Geometry: final body of the model. Coordinates: model frame, mm. A direction names the side the tool comes from. Coordinates: 2 decimals unless noted, no trailing zeros. Write each loop counter-clockwise with the first axis right and the second up, starting at its lowest first coordinate (ties: lowest second). Pieces come first, ordered by that corner, then holes.
from build123d import *

# Parameters (mm, degrees)
BOSS_EXTRUDE1_DEPTH = 2
FILLET1_R           = 0.5
SKETCH2_R           = 9
BOSS_EXTRUDE2_DEPTH = 1
SKETCH3_R           = 8.5
BOSS_EXTRUDE3_DEPTH = 4
CUT_EXTRUDE1_DEPTH  = 16.375249198


with BuildPart() as part:
    # Sketch1 → Boss-Extrude1 (new body)
    with BuildSketch(Plane(origin=(0, 31, 0), x_dir=(1, 0, 0), z_dir=(0, 1, 0))):
        Polygon((0, 10.392304845), (-9, 5.196152423), (-9, -5.196152423), (0, -10.392304845), (9, -5.196152423), (9, 5.196152423), align=None)
    extrude(amount=BOSS_EXTRUDE1_DEPTH)

    # Fillet1
    fillet1_edges = [part.edges().sort_by_distance(p)[0] for p in [
        (9, 32, -5.196152423),
        (9, 32, 5.196152423),
        (0, 32, 10.392304845),
        (-9, 32, 5.196152423),
        (-9, 32, -5.196152423),
        (0, 32, -10.392304845),
    ]]
    fillet(fillet1_edges, radius=FILLET1_R)

    # Sketch2 → Boss-Extrude2 (add)
    with BuildSketch(Plane(origin=(0, 33, 0), x_dir=(1, 0, 0), z_dir=(0, 1, 0))):
        with Locations(Location((0, 0, 0), (0, 0, 60))):
            Circle(SKETCH2_R)
    extrude(amount=BOSS_EXTRUDE2_DEPTH)

    # Sketch3 → Boss-Extrude3 (add)
    with BuildSketch(Plane(origin=(0, 34, 0), x_dir=(1, 0, 0), z_dir=(0, 1, 0))):
        with Locations(Location((0, 0, 0), (0, 0, 270))):
            Circle(SKETCH3_R)
    extrude(amount=BOSS_EXTRUDE3_DEPTH)

    # Sketch4 → Cut-Extrude1 (cut, through all)
    with BuildSketch(Plane(origin=(0, 38, 0), x_dir=(1, 0, 0), z_dir=(0, 1, 0))):
        Polygon((0, 2.886751346), (-2.5, 1.443375673), (-2.5, -1.443375673), (0, -2.886751346), (2.5, -1.443375673), (2.5, 1.443375673), align=None)
    extrude(amount=-CUT_EXTRUDE1_DEPTH, mode=Mode.SUBTRACT)


solid = part.part
Item 1: Section B-B, the plane z = -1. Output: boundary loops of the cut face in (x, y).
Derived:
outline: (-9, 31) - (-2.5, 31) - (-2.5, 38) - (-8.44, 38) - (-8.44, 34) - (-8.94, 34) - (-8.94, 33) - (-9, 33) - close; (2.5, 31) - (9, 31) - (9, 33) - (8.94, 33) - (8.94, 34) - (8.44, 34) - (8.44, 38) - (2.5, 38) - close
Item 2: Section A-A, the plane y = 36.75. Output: boundary loops of the cut face in (x, z).
Derived:
outline: circle Ø17 at (0, 0); hole (-2.5, -1.44) - (0, -2.89) - (2.5, -1.44) - (2.5, 1.44) - (0, 2.89) - (-2.5, 1.44) - close
Item 3: Pull-direction query (X, two-part tool) for faces 5 (the flat face through (1.267, 34.549, -2.155)), 6 (the flat face through (4.56, 31.99, -7.76)), 7 (the cylindrical face through (8.428, 35.972, -1.107)), 8 (the flat face through (-2, 31, 2)); classes: released by +X, released by -X, zero draft, split by the parting line, or undercut.
Derived:
face 5: undercut
face 6: released by +X
face 7: split by the parting line
face 8: zero draft
Item 4: Section C-C, the plane x = -7. Output: boundary loops of the cut face in (y, z), plus the area to 3 significant figures.
Derived:
outline: (31, -6.35) - (33, -6.35) - (33, -5.66) - (34, -5.66) - (34, -4.82) - (38, -4.82) - (38, 4.82) - (34, 4.82) - (34, 5.66) - (33, 5.66) - (33, 6.35) - (31, 6.35) - close
area: 75.3 mm2
Item 5: Section D-D, the plane z = -6.25. Output: boundary loops of the cut face in (x, y).
Derived:
outline: (-7.17, 31) - (7.17, 31) - (7.17, 33) - (6.48, 33) - (6.48, 34) - (5.76, 34) - (5.76, 38) - (-5.76, 38) - (-5.76, 34) - (-6.48, 34) - (-6.48, 33) - (-7.17, 33) - close
Item 6: Set-up query: faces 1 (the flat face through (-8, 33, 5)), 2 (the flat face through (-1.233, 34.549, -2.175)), 3 (the flat face through (8.1, 33, -4.5)), 4 (the flat face through (7.7, 34, -4)). Return all of +Z, -Z, +X, -X, +Y, -Y with unobstructed straight access to the full face (end or side cutting, diameter ignored); none if empty.
Derived:
face 1: +Z, -X, +Y
face 2: +Y, -Y
face 3: -Z, +X, +Y
face 4: +Y
Item 7: Pin query (flat end, axial travel): pin 1 (3 mm diameter, centred on x = -1, z = 9.5, fed in from +Y); pin 2 (1.5 mm diameter, centred on x = -1.5, y = 36, fed in from +Z); pin 3 (4 mm diameter, centred on y = 37, z = 4, fed in from +X); pin 4 (2.5 mm diameter, centred on y = 35.5, z = -0.5, fed in from +X). Return the tip coordinate at first contact, or that it passes through.
Derived:
pin 1: stops at y = 38
pin 2: stops at z = 8.47
pin 3: stops at x = 8.26
pin 4: stops at x = 8.5
Item 8: Material intervals for probe 1 along X at (y, z) = (36, -2.5); probe 2 along Z at (x, y) = (0.5, 34.5); probe 3 along X at (y, z) = (35.5, 1), sorted ascending.
Derived:
probe 1: x = -8.12 to -0.67, 0.67 to 8.12
probe 2: z = -8.49 to -2.6, 2.6 to 8.49
probe 3: x = -8.44 to -2.5, 2.5 to 8.44
